Geometry check sheet. Reference: the model listing, model coordinates, mm. Face numbers are marked on the shaded views. A direction names the side the tool comes from. Round coordinates to 2 decimals unless told otherwise and drop trailing zeros. Write each loop counter-clockwise with the first axis right and the second up, starting at its lowest first coordinate (ties: lowest second). Pieces come first, ordered by that corner, then holes. Notation, with made-up numbers: M 41.25,3 L 83.25,3 A13 cw 83.25,20 Z; hole C -23.75,-10 d6. An arc over 180 degrees is marked long. One line per item, written item: value. Start each with the question number.
1. Depth check by flat-ended pin: P1, Ø6, axis at x = 10.5, y = 1, coming from the -Z side; P2, Ø3, axis at x = -8, z = 5.5, coming from the -Y side; P3, Ø10, axis at x = 3.5, z = -1.5, coming from the +Y side (3 decimals); P4, Ø5, axis at y = 0, z = -11.5, coming from the +X side. Enter the tip coordinate at first touch or a pass-through.
2. Scan lines: probe 1 along X at (y, z) = (0, 13) (3 decimals); probe 2 along X at (y, z) = (0, 9.5) (3 decimals); probe 3 along Z at (x, y) = (6, -0.5). Record each from-to range of solid material in increasing order. Write a range as [from, to].
3. Section check A-A (z = -10.5). Record the boundary of the cut face in (x, y), and give its area (3 significant figures).
4. Access from +Z, -Z, +X, -X, +Y, -Y to the whole of each face (thin tool, end or side, straight path). Record for the marked faces 1 and 2.
5. Section check B-B (y = 13). Record the boundary of the cut face in (x, z), and give its area (3 significant figures).
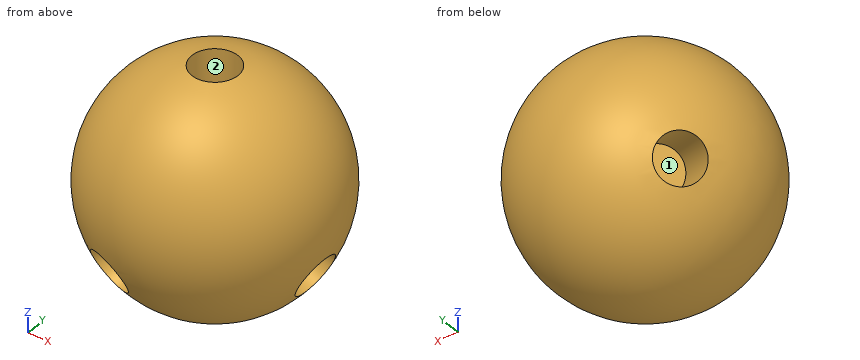
from build123d import *

# Parameters (mm, degrees)
F5_R      = 3.175
F6_DEPTH  = 50.8
F9_ANGLE  = 115.8
F10_ANGLE = 108.4
F11_ANGLE = 107.7


# Not quite as in the source:
# - a length typed as a fraction of an inch, garbled in the dataset ("3 / 203.2 mm" for 3/8 in), is restored


with BuildPart() as f2:
    # F0 (on Front) → F2 (revolve)
    with BuildSketch(Plane.XZ):
        with BuildLine():
            Line((0, -15.875), (0, 15.875))
            ThreePointArc((0, 15.875), (-15.875, 0), (0, -15.875))
        make_face()
    revolve(axis=Axis((0, 0, 0), (0, 0, 1)))


with BuildPart() as f6:
    # F5 (on offset) → F6 (new body)
    with BuildSketch(Plane.XY.offset(5.715)):
        Circle(F5_R)
    extrude(amount=F6_DEPTH)


with BuildPart() as f9_1:
    # F9: copy of F6
    add(f6.part.rotate(Axis((0, 33.8576585054, 0), (0, 1, 0)), F9_ANGLE))


with BuildPart() as f10_1:
    # F10: copy of F9_1
    add(f9_1.part.rotate(Axis((0, 0, -28.0886162072), (0, 0, -1)), F10_ANGLE))


with BuildPart() as f11_1:
    # F11: copy of F10_1
    add(f10_1.part.rotate(Axis((0, 0, -28.0886162072), (0, 0, -1)), F11_ANGLE))


with BuildPart() as f2_1:
    add(f2.part)

    # F12: cut F6, F10_1, F11_1, F9_1
    add(f6.part, mode=Mode.SUBTRACT)
    add(f10_1.part, mode=Mode.SUBTRACT)
    add(f11_1.part, mode=Mode.SUBTRACT)
    add(f9_1.part, mode=Mode.SUBTRACT)


solid = f2_1.part
Result sheet:
1. P1: stops at z = -13.97
1. P2: stops at y = -13.59
1. P3: stops at y = 15.875
1. P4: stops at x = 12.75
2. probe 1: x = [-9.111, -3.175], [3.175, 9.111]
2. probe 2: x = [-12.719, -3.175], [3.175, 12.719]
2. probe 3: z = [-14.69, -6.38], [-0.72, 14.69]
3. outline: C 0,0 d23.81
3. area: 445 mm2
4. face 1: none
4. face 2: +Z
5. outline: C 0,0 d18.22
5. area: 261 mm2
